Design review of the part shown in the three views and the two pictorial views. Dimensions are in mm from the part's minimum x, y and z. A direction names the side the tool comes from. Coordinates: 2 decimals unless noted, no trailing zeros. Order: outer loops, then holes, each group sorted by start corner. A loop starts at its lowest first (then second) coordinate and runs counter-clockwise, first axis right, second up. Notation, with made-up numbers: M 26.5,6.5 L 36.5,6.5 A34 cw 36.5,45.5 Z; hole C 62,-18.5 d2. An arc over 180 degrees is marked long. Use CSV: the item, a comma, the result in double quotes.
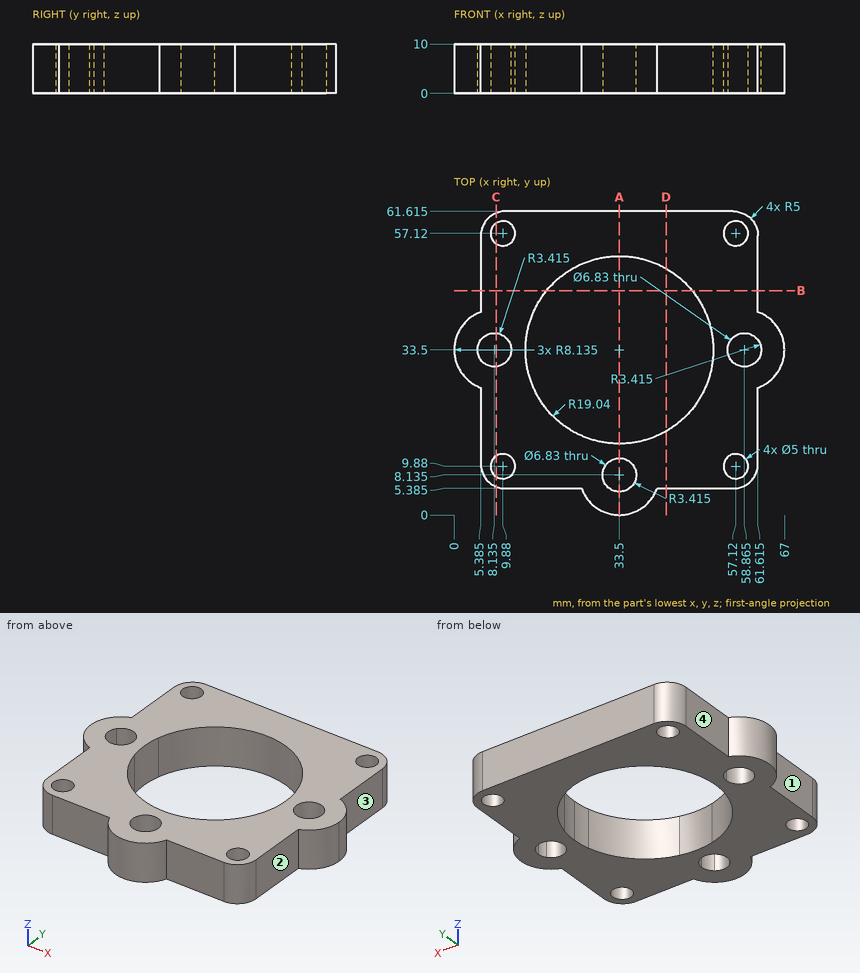
(1) Clearance check with flat-ended pins moving along their axes: P1, Ø6, axis at y = 13, z = 3.5, coming from the +X side (3 decimals); P2, Ø3, axis at x = 9.88, y = 9.88, coming from the +Z side; P3, Ø2, axis at y = 13, z = 4, coming from the -X side (3 decimals); P4, Ø1, axis at x = 7, z = 1.5, coming from the -Y side. State where each tip first meets the part, or that it passes through.
The answers:
P1,"stops at x = 61.615"
P2,"passes through"
P3,"stops at x = 5.385"
P4,"stops at y = 6.3"
(2) For the marked faces 1, 2, 3 and 4, list the 3-axis set-ups (+Z, -Z, +X, -X, +Y, -Y) from which the entire face can be reached by the end or side of a thin tool; tool diameter is ignored.
The answers:
face 1,"+Z, -Z, -X, -Y"
face 2,"+Z, -Z, +X, -Y"
face 3,"+Z, -Z, +X, +Y"
face 4,"+Z, -Z, -X, +Y"
(3) Add section C-C on x = 8.5. State the section outline as (y, z) points.
The answers:
outline,"M 5.75,0 L 7.8,0 L 7.8,10 L 5.75,10 Z; M 11.96,0 L 30.1,0 L 30.1,10 L 11.96,10 Z; M 36.9,0 L 55.04,0 L 55.04,10 L 36.9,10 Z; M 59.2,0 L 61.25,0 L 61.25,10 L 59.2,10 Z"
(4) Add section D-D on x = 43. State the section outline as (y, z) points (3 decimals), and give its area (3 significant figures).
The answers:
outline,"M 5.385,0 L 16.999,0 L 16.999,10 L 5.385,10 Z; M 50.001,0 L 61.615,0 L 61.615,10 L 50.001,10 Z"
area,"232 mm2"
(5) Wall thickness on probe 1 along Y at (x, z) = (33.5, 3.5) (3 decimals); probe 2 along X at (y, z) = (57, 6.5); probe 3 along Y at (x, z) = (56, 4.5) (1 decimal): over which ranges is each line inside the solid? List them lowest first.
The answers:
probe 1,"y = 0 to 4.72, 11.55 to 14.46, 52.54 to 61.615"
probe 2,"x = 5.4 to 7.38, 12.38 to 54.62, 59.62 to 61.6"
probe 3,"y = 5.4 to 7.6, 12.1 to 31.6, 35.4 to 54.9, 59.4 to 61.6"
(6) Add section A-A on x = 33.5. State the section outline as (y, z) points (3 decimals).
The answers:
outline,"M 0,0 L 4.72,0 L 4.72,10 L 0,10 Z; M 11.55,0 L 14.46,0 L 14.46,10 L 11.55,10 Z; M 52.54,0 L 61.615,0 L 61.615,10 L 52.54,10 Z"
(7) Add section B-B on y = 45.5. State the section outline as (x, z) points (3 decimals), and give its area (3 significant figures).
The answers:
outline,"M 5.385,0 L 18.718,0 L 18.718,10 L 5.385,10 Z; M 48.282,0 L 61.615,0 L 61.615,10 L 48.282,10 Z"
area,"267 mm2"
